```python
from build123d import *

# Parameters (mm, degrees)
SKETCH_1_R         = 30
SKETCH_1_R_2       = 1.5
SKETCH_1_R_3       = 2
SKETCH_1_W         = 120
SKETCH_1_H         = 120
EXTRUDE_1_DEPTH    = 4
HOLE_WIZARD_M4_1_D = 3.3
HOLE_WIZARD_M5_1_D = 4.2


with BuildPart() as part:
    # 草图1 → 凸台-拉伸1 (new body)
    with BuildSketch(Plane.XY):
        with BuildLine():
            Line((-140, 50), (-140, -50))
            Line((-140, -50), (-152, -50))
            ThreePointArc((-152, -50), (-157.656854249, -52.343145751), (-160, -58))
            Line((-160, -58), (-160, -170))
            ThreePointArc((-160, -170), (-151.213203436, -191.213203436), (-130, -200))
            Line((-130, -200), (130, -200))
            ThreePointArc((130, -200), (151.213203436, -191.213203436), (160, -170))
            Line((160, -170), (160, -58))
            ThreePointArc((160, -58), (157.656854249, -52.343145751), (152, -50))
            Line((152, -50), (140, -50))
            Line((140, -50), (140, 50))
            Line((140, 50), (152, 50))
            ThreePointArc((152, 50), (157.656854249, 52.343145751), (160, 58))
            Line((160, 58), (160, 170))
            ThreePointArc((160, 170), (151.213203436, 191.213203436), (130, 200))
            Line((130, 200), (-130, 200))
            ThreePointArc((-130, 200), (-151.213203436, 191.213203436), (-160, 170))
            Line((-160, 170), (-160, 58))
            ThreePointArc((-160, 58), (-157.656854249, 52.343145751), (-152, 50))
            Line((-152, 50), (-140, 50))
        make_face()
        with Locations((-120, 160)):
            Circle(SKETCH_1_R, mode=Mode.SUBTRACT)
        with Locations((120, 160)):
            Circle(SKETCH_1_R, mode=Mode.SUBTRACT)
        with Locations((-120, -160.002034224)):
            Circle(SKETCH_1_R, mode=Mode.SUBTRACT)
        with Locations((120, -160.002034224)):
            Circle(SKETCH_1_R, mode=Mode.SUBTRACT)
        with Locations((-120, 195)):
            Circle(SKETCH_1_R_2, mode=Mode.SUBTRACT)
        with Locations((-155, 160)):
            Circle(SKETCH_1_R_2, mode=Mode.SUBTRACT)
        with Locations((-120, 125)):
            Circle(SKETCH_1_R_2, mode=Mode.SUBTRACT)
        with Locations((-85, 160)):
            Circle(SKETCH_1_R_2, mode=Mode.SUBTRACT)
        with Locations((120, 195)):
            Circle(SKETCH_1_R_2, mode=Mode.SUBTRACT)
        with Locations((155, 160)):
            Circle(SKETCH_1_R_2, mode=Mode.SUBTRACT)
        with Locations((85, 160)):
            Circle(SKETCH_1_R_2, mode=Mode.SUBTRACT)
        with Locations((120, 125)):
            Circle(SKETCH_1_R_2, mode=Mode.SUBTRACT)
        with Locations((-155, -160.002034224)):
            Circle(SKETCH_1_R_2, mode=Mode.SUBTRACT)
        with Locations((-120, -195.002034224)):
            Circle(SKETCH_1_R_2, mode=Mode.SUBTRACT)
        with Locations((-120, -125.002034224)):
            Circle(SKETCH_1_R_2, mode=Mode.SUBTRACT)
        with Locations((-85, -160.002034224)):
            Circle(SKETCH_1_R_2, mode=Mode.SUBTRACT)
        with Locations((155, -160.002034224)):
            Circle(SKETCH_1_R_2, mode=Mode.SUBTRACT)
        with Locations((120, -195.002034224)):
            Circle(SKETCH_1_R_2, mode=Mode.SUBTRACT)
        with Locations((120, -125.002034224)):
            Circle(SKETCH_1_R_2, mode=Mode.SUBTRACT)
        with Locations((85, -160.002034224)):
            Circle(SKETCH_1_R_2, mode=Mode.SUBTRACT)
        with Locations((25, -100)):
            Circle(SKETCH_1_R_3, mode=Mode.SUBTRACT)
        with Locations((25, -70)):
            Circle(SKETCH_1_R_3, mode=Mode.SUBTRACT)
        with Locations((-25, -100)):
            Circle(SKETCH_1_R_3, mode=Mode.SUBTRACT)
        with Locations((-25, -70)):
            Circle(SKETCH_1_R_3, mode=Mode.SUBTRACT)
        with Locations((-25, 68.76)):
            Circle(SKETCH_1_R_3, mode=Mode.SUBTRACT)
        with Locations((25, 68.76)):
            Circle(SKETCH_1_R_3, mode=Mode.SUBTRACT)
        with Locations((-120, 110)):
            Circle(SKETCH_1_R_3, mode=Mode.SUBTRACT)
        with Locations((120, 110)):
            Circle(SKETCH_1_R_3, mode=Mode.SUBTRACT)
        with Locations((-70, -160.002034224)):
            Circle(SKETCH_1_R_3, mode=Mode.SUBTRACT)
        with Locations((70, -160.002034224)):
            Circle(SKETCH_1_R_3, mode=Mode.SUBTRACT)
        with Locations((-126.75, 9.3)):
            Circle(SKETCH_1_R_3, mode=Mode.SUBTRACT)
        with Locations((-111.25, 9.3)):
            Circle(SKETCH_1_R_3, mode=Mode.SUBTRACT)
        with Locations((-126.75, -26.7)):
            Circle(SKETCH_1_R_3, mode=Mode.SUBTRACT)
        with Locations((-111.25, -26.7)):
            Circle(SKETCH_1_R_3, mode=Mode.SUBTRACT)
        with Locations((111.25, 9.3)):
            Circle(SKETCH_1_R_3, mode=Mode.SUBTRACT)
        with Locations((126.75, 9.3)):
            Circle(SKETCH_1_R_3, mode=Mode.SUBTRACT)
        with Locations((111.25, -26.7)):
            Circle(SKETCH_1_R_3, mode=Mode.SUBTRACT)
        with Locations((126.75, -26.7)):
            Circle(SKETCH_1_R_3, mode=Mode.SUBTRACT)
        Rectangle(SKETCH_1_W, SKETCH_1_H, mode=Mode.SUBTRACT)
        with BuildLine():
            Line((-52.5, 170), (-52.5, 142))
            ThreePointArc((-52.5, 142), (-55, 139.5), (-57.5, 142))
            Line((-57.5, 142), (-57.5, 170))
            ThreePointArc((-57.5, 170), (-55, 172.5), (-52.5, 170))
        make_face(mode=Mode.SUBTRACT)
        with BuildLine():
            Line((-52.5, 123), (-52.5, 95))
            ThreePointArc((-52.5, 95), (-55, 92.5), (-57.5, 95))
            Line((-57.5, 95), (-57.5, 123))
            ThreePointArc((-57.5, 123), (-55, 125.5), (-52.5, 123))
        make_face(mode=Mode.SUBTRACT)
        with BuildLine():
            Line((57.5, 170), (57.5, 142))
            ThreePointArc((57.5, 142), (55, 139.5), (52.5, 142))
            Line((52.5, 142), (52.5, 170))
            ThreePointArc((52.5, 170), (55, 172.5), (57.5, 170))
        make_face(mode=Mode.SUBTRACT)
        with BuildLine():
            Line((57.5, 123), (57.5, 95))
            ThreePointArc((57.5, 95), (55, 92.5), (52.5, 95))
            Line((52.5, 95), (52.5, 123))
            ThreePointArc((52.5, 123), (55, 125.5), (57.5, 123))
        make_face(mode=Mode.SUBTRACT)
    extrude(amount=EXTRUDE_1_DEPTH)

    # M4 螺纹孔1 (through all)
    with Locations(Plane.XY.offset(4)):
        with Locations((-120, 195), (-155, 160), (-85, 160), (-120, 125), (120, 195), (85, 160), (120, 125), (155, 160), (-120, -125.002034224), (-155, -160.002034224), (-85, -160.002034224), (-120, -195.002034224), (120, -125.002034224), (85, -160.002034224), (155, -160.002034224), (120, -195.002034224)):
            Hole(HOLE_WIZARD_M4_1_D / 2)

    # M5 螺纹孔1 (through all)
    with Locations(Plane.XY.offset(4)):
        with Locations((-120, 110), (-25, 68.76), (25, 68.76), (120, 110), (-25, -70), (25, -70), (25, -100), (-25, -100), (-70, -160.002034224), (70, -160.002034224), (-126.75, 9.3), (-111.25, 9.3), (-126.75, -26.7), (-111.25, -26.7), (111.25, 9.3), (126.75, 9.3), (111.25, -26.7), (126.75, -26.7)):
            Hole(HOLE_WIZARD_M5_1_D / 2)


solid = part.part
```
The model under review builds one solid part; all positions refer to its coordinate system, in mm. A direction names the side the tool comes from. Round coordinates to 2 decimals unless told otherwise and drop trailing zeros. Loops run counter-clockwise (first coordinate to the right, second up) from the corner with the lowest first, then second, coordinate; pieces in that order, holes last. Notation, with made-up numbers: M -29.5,3 L -17.5,3 A25 cw -17.5,39 Z; hole C 46.25,-8.5 d2. An arc over 180 degrees is marked long. Put each result on its own line as item: value.
Q1. To check wall thickness, follow L1, parallel to X at y = 98.5, z = 0.9; L2, parallel to X at y = 68.5, z = 2.3; L3, parallel to X at y = -48, z = 3.55. State the ranges of each line that lie inside material, in increasing order.
Result set:
L1: x = -160 to -57.5, -52.5 to 52.5, 57.5 to 160
L2: x = -160 to -27.08, -22.92 to 22.92, 27.08 to 160
L3: x = -140 to -60, 60 to 140
Q2. Consider section A-A, the plane y = 103.5. Give the boundary of the cut face in (x, z).
Result set:
outline: M -160,0 L -57.5,0 L -57.5,4 L -160,4 Z; M -52.5,0 L 52.5,0 L 52.5,4 L -52.5,4 Z; M 57.5,0 L 160,0 L 160,4 L 57.5,4 Z
Q3. Consider section B-B, the plane z = 0.95. Count the separate pieces of the cut face and the enclosed holes in it, then the cut area to 3 significant figures.
Result set:
separate pieces: 1
enclosed holes: 43
area: 96,400 mm²
Q4. Mouldability with a two-part tool opening along Y and no side actions: class faces 4 (the flat face through (69, 3, 0)), 5 (the cylindrical face through (150.979, -191.445, 1.972)), 6 (the cylindrical face through (-157.594, -52.281, 1.972)), 7 (the cylindrical face through (151.445, 190.979, 1.972)) as released by +Y, released by -Y, zero draft, split by the parting line, or undercut.
Result set:
face 4: zero draft
face 5: released by -Y
face 6: undercut
face 7: released by +Y
Q5. Machinability: for faces 1 (the cylindrical face through (-126.503, 130.713, 1.972)), 2 (the cylindrical face through (-157.719, 52.406, 1.972)), 3 (the cylindrical face through (157.719, -52.406, 1.972)), which of the approach directions +Z, -Z, +X, -X, +Y, -Y give a long, thin tool a straight path to every point of the face, cutting with its end or side? Answer none if there is none.
Result set:
face 1: +Z, -Z
face 2: +Z, -Z, -X
face 3: +Z, -Z, +X
Q6. For pin 1 (4.5 mm diameter, centred on x = 85, y = 160, fed in from +Z), flat-tipped, find the tip position at first contact; note if it passes through.
Result set:
pin 1: stops at z = 4
